Verification items for this drawing (mm, ordinates from the low corner). Give positions to 0.01 mm unless a question says otherwise; leave off trailing zeros. Order: outer loops, then holes, each group sorted by start corner. A loop starts at its lowest first (then second) coordinate and runs counter-clockwise, first axis right, second up.
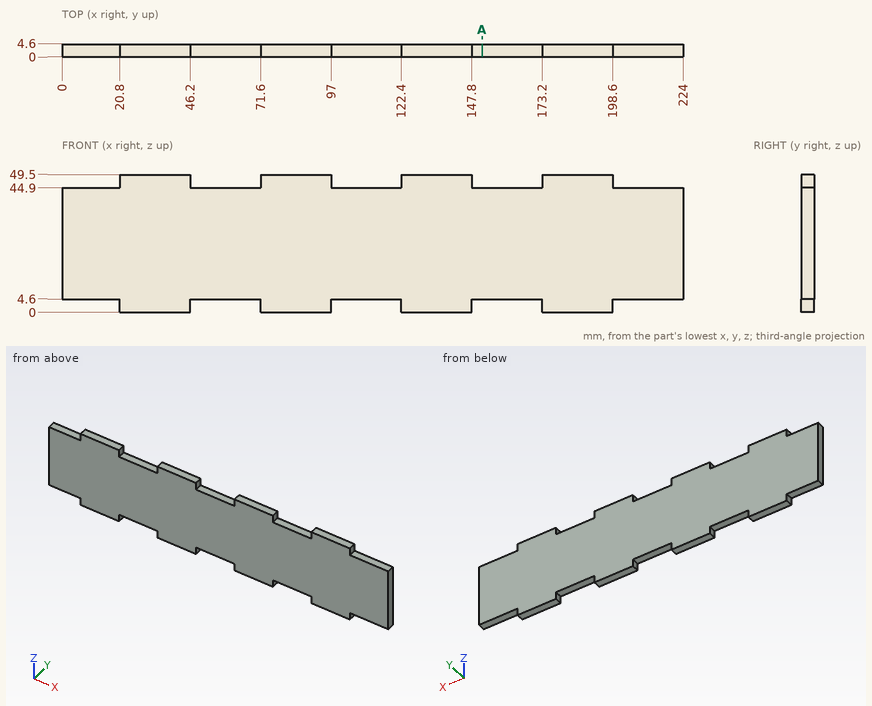
Q1. Thickness scan on L1, parallel to X at y = 4.3, z = 4; L2, parallel to Z at x = 169, y = 3.9. Record the ranges inside material, lowest first.
Q2. Gauge pin test, flat ends, axial feed: P1, Ø2.5, axis at y = 2.5, z = 48, coming from the +X side; P2, Ø1.4, axis at y = 3.5, z = 47, coming from the -X side; P3, Ø2.5, axis at x = 55.5, y = 1.5, coming from the +Z side. Record the tip position at first contact, or that the pin passes through.
Q3. Cross-section at A-A, the plane x = 151.5. Record the boundary of the cut face in (y, z), and give its area (3 significant figures).
Answers follow:
1. L1: x = 20.8 to 46.2, 71.6 to 97, 122.4 to 147.8, 173.2 to 198.6
1. L2: z = 4.6 to 44.9
2. P1: stops at x = 198.6
2. P2: stops at x = 20.8
2. P3: stops at z = 44.9
3. outline: (0, 4.6) - (4.6, 4.6) - (4.6, 44.9) - (0, 44.9) - close
3. area: 185 mm2
